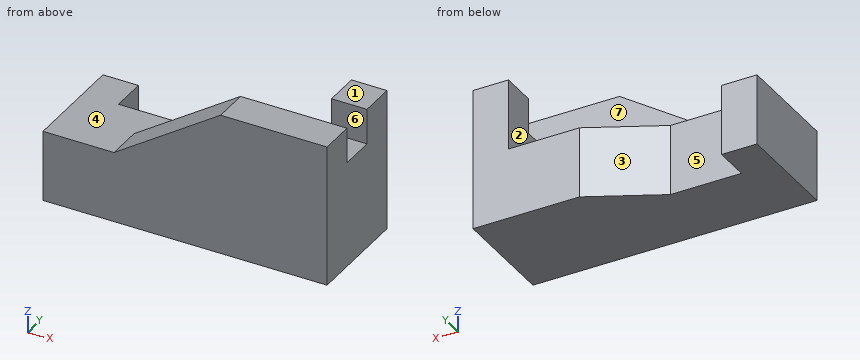
```python
from build123d import *

# Parameters (mm, degrees)
BOSS_EXTRUDE1_DEPTH = 20
SKETCH2_W           = 30
SKETCH2_H           = 10
BOSS_EXTRUDE2_DEPTH = 20
BOSS_EXTRUDE3_DEPTH = 10
SKETCH4_W           = 10
SKETCH4_H           = 20
BOSS_EXTRUDE4_DEPTH = 10
SKETCH5_W           = 10
SKETCH5_H           = 10
BOSS_EXTRUDE5_DEPTH = 10


with BuildPart() as part:
    # Sketch1 → Boss-Extrude1 (new body)
    with BuildSketch(Plane.XY):
        Polygon((-29.033595627, 12.701314612), (-29.033595627, 2.701314612), (-9.033595627, 2.701314612), (10.966404373, 12.701314612), (40.966404373, 12.701314612), (40.966404373, -17.298685388), (-39.033595627, -17.298685388), (-39.033595627, 12.701314612), align=None)
    extrude(amount=BOSS_EXTRUDE1_DEPTH)

    # Sketch2 → Boss-Extrude2 (add)
    with BuildSketch(Plane.XY.offset(20)):
        with Locations((25.966404373, -12.298685388)):
            Rectangle(SKETCH2_W, SKETCH2_H)
    extrude(amount=BOSS_EXTRUDE2_DEPTH)

    # Sketch3 → Boss-Extrude3 (add)
    with BuildSketch(Plane(origin=(0, -17.298685388, 0), x_dir=(-1, 0, 0), z_dir=(0, -1, 0))):
        Polygon((-10.966404373, -40), (19.033595627, -20), (-10.966404373, -20), align=None)
    extrude(amount=-BOSS_EXTRUDE3_DEPTH)

    # Sketch4 → Boss-Extrude4 (add)
    with BuildSketch(Plane.XY.offset(20)):
        with Locations((35.966404373, 2.701314612)):
            Rectangle(SKETCH4_W, SKETCH4_H)
    extrude(amount=BOSS_EXTRUDE4_DEPTH)

    # Sketch5 → Boss-Extrude5 (add)
    with BuildSketch(Plane.XY.offset(30)):
        with Locations((35.966404373, 7.701314612)):
            Rectangle(SKETCH5_W, SKETCH5_H)
    extrude(amount=BOSS_EXTRUDE5_DEPTH)


solid = part.part
```
The listing builds one solid part. Answer for the finished solid, in the listing's coordinates (mm). Face numbers are marked on the shaded views. A direction names the side the tool comes from. Give positions to 0.01 mm unless a question says otherwise; leave off trailing zeros. Write each loop counter-clockwise with the first axis right and the second up, starting at its lowest first coordinate (ties: lowest second). Pieces come first, ordered by that corner, then holes. Notation, with made-up numbers: M 88.25,4 L 140.25,4 A36 ccw 140.25,39 Z; hole C 23,32 d8. An arc over 180 degrees is marked long. Write each question's results on one line, items separated by ' | '.
Q1. For a pull along X with two mould halves and no side action, classify the marked faces 1, 2 and 3 as released by +X, released by -X, zero draft, split by the parting line, or undercut.
Output values:
face 1: zero draft | face 2: released by -X | face 3: undercut
Q2. Section A-A, the plane y = 9 is taken. Write down the section's boundary in (x, z).
Output values:
outline: M -39.03,0 L -29.03,0 L -29.03,20 L -39.03,20 Z; M 3.56,0 L 40.97,0 L 40.97,40 L 30.97,40 L 30.97,20 L 3.56,20 Z
Q3. Section C-C, the plane x = 14.5 is taken. Write down the section's boundary in (y, z).
Output values:
outline: M -17.3,0 L 12.7,0 L 12.7,20 L -7.3,20 L -7.3,40 L -17.3,40 Z
Q4. Section B-B, the plane z = 34 is taken. Write down the section's boundary in (x, y), then the cut area to 3 significant figures.
Output values:
outline: M 1.97,-17.3 L 40.97,-17.3 L 40.97,-7.3 L 1.97,-7.3 Z; M 30.97,2.7 L 40.97,2.7 L 40.97,12.7 L 30.97,12.7 Z | area: 490 mm2
Q5. Section D-D, the plane z = 15 is taken. Write down the section's boundary in (x, y).
Output values:
outline: M -39.03,-17.3 L 40.97,-17.3 L 40.97,12.7 L 10.97,12.7 L -9.03,2.7 L -29.03,2.7 L -29.03,12.7 L -39.03,12.7 Z
Q6. Flat-ended cylindrical pins translate along their axes: P1, Ø3, axis at y = 7.5, z = 24.5, coming from the -X side; P2, Ø6, axis at x = -21, z = 7.5, coming from the +Y side; P3, Ø10, axis at x = -29, y = -7, coming from the +Z side; P4, Ø6, axis at x = 14, y = 7.5, coming from the -Z side. Find the tip coordinate at first contact, or state that the pin passes through.
Output values:
P1: x = 30.97 | P2: y = 2.7 | P3: z = 20 | P4: z = 0
Q7. Consider L1, parallel to Z at x = -17, y = -3; L2, parallel to Z at x = 32, y = -4.5; L3, parallel to X at y = 7, z = 29.5. Determine where each line is inside the solid, lowest interval first. Write a range as from..to.
Output values:
L1: 0..20 | L2: 0..30 | L3: 30.97..40.97
Q8. A tool of negligible diameter and unlimited length cuts with its end or side. For the marked faces 4, 5, 6 and 7, from which of +Z, -Z, +X, -X, +Y, -Y can it reach the whole face along a straight path? Write none if from no direction.
Output values:
face 4: +Z, -X, +Y | face 5: +Z, -Z, +Y | face 6: +Z, +X, -X | face 7: +Z, -X
